Part model, mm, in its own coordinate system. Coordinates: 2 decimals unless noted, no trailing zeros. Order: outer loops, then holes, each group sorted by start corner. A loop starts at its lowest first (then second) coordinate and runs counter-clockwise, first axis right, second up.
```python
from build123d import *

# Parameters (mm, degrees)
SKETCH1_R           = 141.421356237
SKETCH1_W           = 25.4
SKETCH1_H           = 25.4
BOSS_EXTRUDE1_DEPTH = 5


with BuildPart() as part:
    # Sketch1 → Boss-Extrude1 (new body)
    with BuildSketch(Plane(origin=(0, 0, 0), x_dir=(1, 0, 0), z_dir=(0, 1, 0))):
        with BuildLine():
            Line((115, 165.4), (110, 165.4))
            Line((110, 165.4), (110, 190.525588833))
            ThreePointArc((110, 190.525588833), (0, 220), (-110, 190.525588833))
            Line((-110, 190.525588833), (-110, 165.4))
            Line((-110, 165.4), (-115, 165.4))
            Line((-115, 165.4), (-115, 187.549993335))
            ThreePointArc((-115, 187.549993335), (-155.563491861, 155.563491861), (-187.549993335, 115))
            Line((-187.549993335, 115), (-165.4, 115))
            Line((-165.4, 115), (-165.4, 110))
            Line((-165.4, 110), (-190.525588833, 110))
            ThreePointArc((-190.525588833, 110), (-220, 0), (-190.525588833, -110))
            Line((-190.525588833, -110), (-165.4, -110))
            Line((-165.4, -110), (-165.4, -115))
            Line((-165.4, -115), (-187.549993335, -115))
            ThreePointArc((-187.549993335, -115), (-155.563491861, -155.563491861), (-115, -187.549993335))
            Line((-115, -187.549993335), (-115, -165.4))
            Line((-115, -165.4), (-110, -165.4))
            Line((-110, -165.4), (-110, -190.525588833))
            ThreePointArc((-110, -190.525588833), (0, -220), (110, -190.525588833))
            Line((110, -190.525588833), (110, -165.4))
            Line((110, -165.4), (115, -165.4))
            Line((115, -165.4), (115, -187.549993335))
            ThreePointArc((115, -187.549993335), (155.563491861, -155.563491861), (187.549993335, -115))
            Line((187.549993335, -115), (165.4, -115))
            Line((165.4, -115), (165.4, -110))
            Line((165.4, -110), (190.525588833, -110))
            ThreePointArc((190.525588833, -110), (220, 0), (190.525588833, 110))
            Line((190.525588833, 110), (165.4, 110))
            Line((165.4, 110), (165.4, 115))
            Line((165.4, 115), (187.549993335, 115))
            ThreePointArc((187.549993335, 115), (155.563491861, 155.563491861), (115, 187.549993335))
            Line((115, 187.549993335), (115, 165.4))
        make_face()
        with Locations(Location((0, 0, 0), (0, 0, 270))):
            Circle(SKETCH1_R, mode=Mode.SUBTRACT)
        with Locations((127.7, 127.7)):
            Rectangle(SKETCH1_W, SKETCH1_H, mode=Mode.SUBTRACT)
        with Locations((-127.7, 127.7)):
            Rectangle(SKETCH1_W, SKETCH1_H, mode=Mode.SUBTRACT)
        with Locations((127.7, -127.7)):
            Rectangle(SKETCH1_W, SKETCH1_H, mode=Mode.SUBTRACT)
        with Locations((-127.7, -127.7)):
            Rectangle(SKETCH1_W, SKETCH1_H, mode=Mode.SUBTRACT)
    extrude(amount=BOSS_EXTRUDE1_DEPTH)


solid = part.part
```
(1) Slice it at B-B, the plane x = 0. Give the cut face in (y, z).
(2) Pull direction X, two halves, no side cores. Call faces 1 (the face through (-219.994, 2.465, -1.613)), 2 (the face through (42.48, 2.46, 134.89)), 3 (the face through (156.075, 2.465, -155.05)), 4 (the face through (-3, 0, 144)): +X half, -X half, draft (parallel to the pull), parting line (faces both ways), or undercut.
(3) Drop flat-ended pins along their axis: pin 1 (2.5 mm diameter, centred on x = -122, y = 1.5, fed in from -Z); pin 2 (2.5 mm diameter, centred on y = 3, z = 175.5, fed in from -X); pin 3 (2.5 mm diameter, centred on x = 126.5, y = 2.5, fed in from -Z). Give the stop position or say it passes through.
(4) Slice it at D-D, the plane z = 131. Give the cut face in (x, y), then the cut area to 3 significant figures.
(5) Probe line 1 (Z direction, x = -171.5, y = 2.85); line 2 (X direction, y = 1.6, z = 0); line 3 (X direction, y = 0.7, z = -172). List the from-to ranges inside material, lowest first.
(6) Slice it at A-A, the plane z = 0. Give the cut face in (x, y), then the cut area to 3 significant figures.
(7) Slice it at C-C, the plane y = 0.9. State how many separate pieces and enclosed holes the cut face has, then the cut area to 3 significant figures.
Here are the results:
1. outline: (0, -220) - (5, -220) - (5, -141.42) - (0, -141.42) - close; (0, 141.42) - (5, 141.42) - (5, 220) - (0, 220) - close
2. face 1: -X half
2. face 2: undercut
2. face 3: +X half
2. face 4: draft
3. pin 1: stops at z = -183.9
3. pin 2: stops at x = -134.3
3. pin 3: stops at z = -180.87
4. outline: (-176.75, 0) - (-140.4, 0) - (-140.4, 5) - (-176.75, 5) - close; (-115, 0) - (-53.28, 0) - (-53.28, 5) - (-115, 5) - close; (53.28, 0) - (115, 0) - (115, 5) - (53.28, 5) - close; (140.4, 0) - (176.75, 0) - (176.75, 5) - (140.4, 5) - close
4. area: 981 mm2
5. line 1: z = -137.8 to -115, -110 to 110, 115 to 137.8
5. line 2: x = -220 to -141.42, 141.42 to 220
5. line 3: x = -137.17 to -115, -110 to 110, 115 to 137.17
6. outline: (-220, 0) - (-141.42, 0) - (-141.42, 5) - (-220, 5) - close; (141.42, 0) - (220, 0) - (220, 5) - (141.42, 5) - close
6. area: 786 mm2
7. separate pieces: 1
7. enclosed holes: 5
7. area: 85,700 mm2
